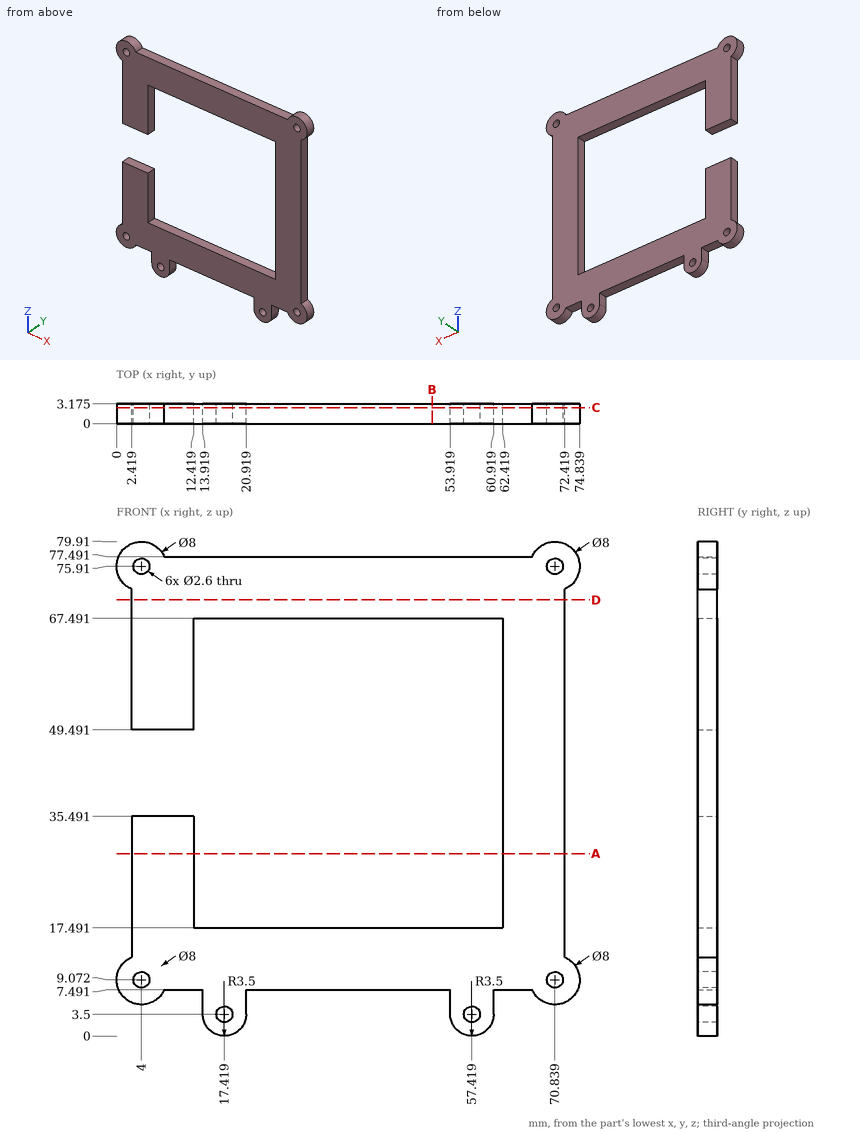
Can you work these out from the drawing? Everything is in mm from the part's minimum corner. Coordinates: 2 decimals unless noted, no trailing zeros. Loops run counter-clockwise (first coordinate to the right, second up) from the corner with the lowest first, then second, coordinate; pieces in that order, holes last. Notation, with made-up numbers: (-15.75, -30) - (31.25, -30) arc R34 ccw to (31.25, 0) - close; hole circle Ø7 at (-26.75, 86.25). An arc over 180 degrees is marked (long way). Put each result on its own line as item: value. Start each with the question number.
Item 1: Suppose I cut it at B-B (x = 51). Please give me the cut outline in (y, z) (1 decimal).
Item 2: Suppose I cut it at A-A (z = 29.5). Please give me the cut outline in (x, y) (1 decimal).
Item 3: Suppose I cut it at D-D (z = 70.5). Please give me the cut outline in (x, y) (1 decimal).
Item 4: Suppose I cut it at C-C (y = 2.6). State how many separate pieces and enclosed holes the cut face has, and give its area (3 significant figures).
Item 5: For pin 1 (3.5 mm diameter, centred on x = 17.42, z = 3.5, fed in from +Y) (1 decimal); pin 2 (1.6 mm diameter, centred on x = 10, y = 1.5, fed in from -Z); pin 3 (1.6 mm diameter, centred on y = 1, z = 57, fed in from +X), each with a flat end and sliding along its axis, tell me the tip position at first contact or that it passes through.
Item 6: If I drill on line 1 along X through (y, z) = (1, 25.5); line 2 along Z through (x, y) = (27.5, 0.8); line 3 along X through (y, z) = (0.7, 76.5) (1 decimal), over which ranges is the centre line in solid material (lowest first)?
Here are the results:
1. outline: (0, 7.5) - (3.2, 7.5) - (3.2, 17.5) - (0, 17.5) - close; (0, 67.5) - (3.2, 67.5) - (3.2, 77.5) - (0, 77.5) - close
2. outline: (2.4, 0) - (12.4, 0) - (12.4, 3.2) - (2.4, 3.2) - close; (62.4, 0) - (72.4, 0) - (72.4, 3.2) - (62.4, 3.2) - close
3. outline: (2.4, 0) - (72.4, 0) - (72.4, 3.2) - (2.4, 3.2) - close
4. separate pieces: 1
4. enclosed holes: 6
4. area: 2,410 mm²
5. pin 1: y = 3.2
5. pin 2: z = 7.49
5. pin 3: x = 72.42
6. line 1: 2.42 to 12.42, 62.42 to 72.42
6. line 2: 7.49 to 17.49, 67.49 to 77.49
6. line 3: 0 to 2.8, 5.2 to 69.7, 72 to 74.8
